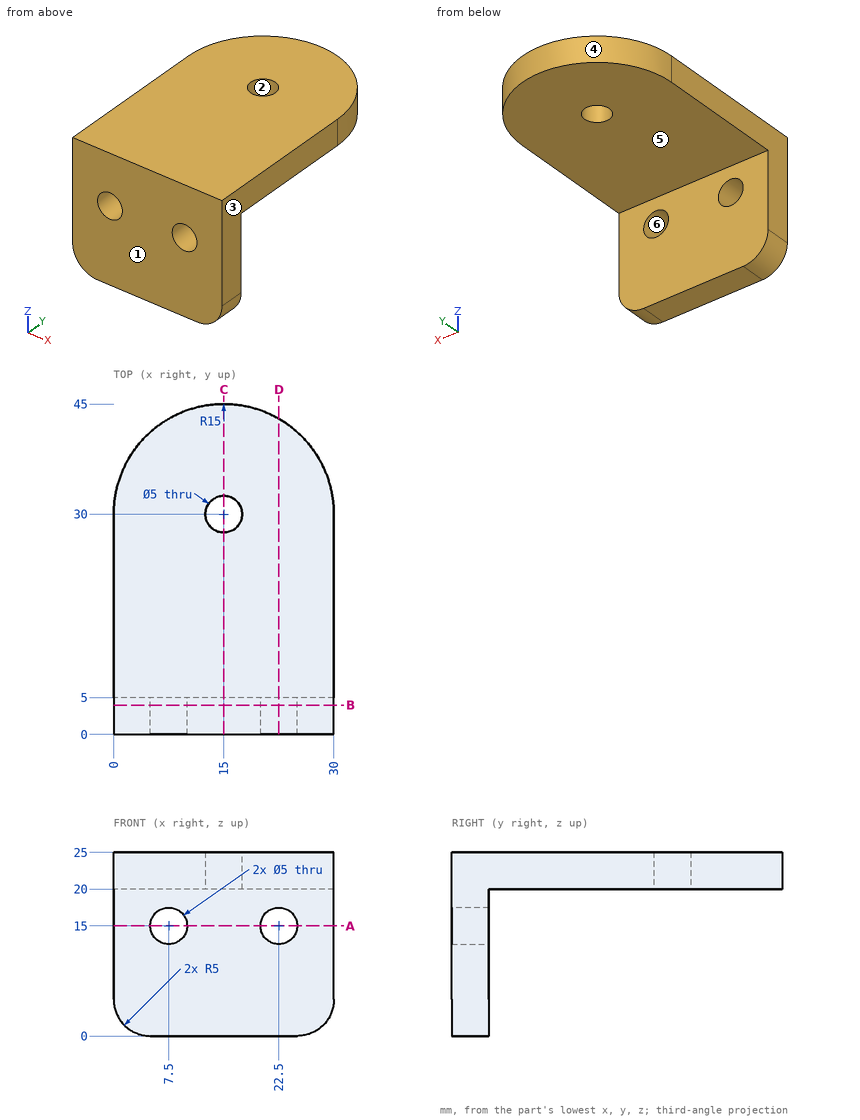
Here's the drawing with two shaded views (mm, measured from the low corner). I have some questions. A direction names the side the tool comes from. Give positions to 0.01 mm unless a question says otherwise; leave off trailing zeros. Write each loop counter-clockwise with the first axis right and the second up, starting at its lowest first coordinate (ties: lowest second). Pieces come first, ordered by that corner, then holes. Notation, with made-up numbers: (-18, 12.25) -> (30, 12.25) arc R23 cw to (30, 48.25) -> close; hole circle Ø8 at (55.5, -33.75). An arc over 180 degrees is marked (long way). Answer as a JSON object with one key per item and string values. Group by question number.
Item 1: For the marked faces 5 and 6, which set-ups out of +Z, -Z, +X, -X, +Y, -Y let a thin tool reach every point of the face, with its end or its side?
Item 2: Suppose I cut it at B-B (y = 4). Please give me the cut outline in (x, z).
Item 3: I'm going to push flat-ended pins straight in: P1, Ø5, axis at x = 21.5, z = 13, coming from the +Y side; P2, Ø10, axis at y = 35.5, z = 20, coming from the -X side; P3, Ø12, axis at x = 20, z = 18.5, coming from the -Y side; P4, Ø10, axis at x = 12, y = 21.5, coming from the -Z side. Where does each tip first touch, or does it pass through?
Item 4: Please list where these lines run through material, in increasing order: line 1 (X direction, y = 1.2, z = 15); line 2 (Y direction, x = 15, z = 23.3); line 3 (X direction, y = 30, z = 23.95). Write a range as [from, to].
Item 5: Suppose I cut it at C-C (x = 15). Please give me the cut outline in (y, z).
Item 6: We'd pull the mould along Y, two halves only. Please class the marked faces 1, 2, 3 and 4: +Y half, -Y half, draft (parallel to the pull), parting line (faces both ways), or undercut.
Item 7: Suppose I cut it at D-D (x = 22.5). Please give me the cut outline in (y, z), plus the area to 3 significant figures.
Item 8: Suppose I cut it at A-A (z = 15). Please give me the cut outline in (x, y), plus the area to 3 significant figures.
Findings:
{
 "1": {"face 5": "-Z, +X, -X, +Y", "face 6": "+Y, -Y"},
 "2": {"outline": "(0, 5) arc R5 ccw to (5, 0) -> (25, 0) arc R5 ccw to (30, 5) -> (30, 25) -> (0, 25) -> close; hole circle Ø5 at (7.5, 15); hole circle Ø5 at (22.5, 15)"},
 "3": {"P1": "stops at y = 5", "P2": "stops at x = 0.01", "P3": "stops at y = 0", "P4": "stops at z = 20"},
 "4": {"line 1": "x = [0, 5], [10, 20], [25, 30]", "line 2": "y = [0, 27.5], [32.5, 45]", "line 3": "x = [0, 12.5], [17.5, 30]"},
 "5": {"outline": "(0, 0) -> (5, 0) -> (5, 20) -> (27.5, 20) -> (27.5, 25) -> (0, 25) -> close; (32.5, 20) -> (45, 20) -> (45, 25) -> (32.5, 25) -> close"},
 "6": {"face 1": "-Y half", "face 2": "undercut", "face 3": "draft", "face 4": "+Y half"},
 "7": {"outline": "(0, 0) -> (5, 0) -> (5, 12.5) -> (0, 12.5) -> close; (0, 17.5) -> (5, 17.5) -> (5, 20) -> (42.99, 20) -> (42.99, 25) -> (0, 25) -> close", "area": "290 mm²"},
 "8": {"outline": "(0, 0) -> (5, 0) -> (5, 5) -> (0, 5) -> close; (10, 0) -> (20, 0) -> (20, 5) -> (10, 5) -> close; (25, 0) -> (30, 0) -> (30, 5) -> (25, 5) -> close", "area": "100 mm²"}
}
